The model under review builds one solid part; all positions refer to its coordinate system, in mm. A direction names the side the tool comes from. Round coordinates to 2 decimals unless told otherwise and drop trailing zeros. Write each loop counter-clockwise with the first axis right and the second up, starting at its lowest first coordinate (ties: lowest second). Pieces come first, ordered by that corner, then holes. Notation, with made-up numbers: (81, -20) - (103, -20) arc R11 cw to (103, -6) - close; hole circle Ø9 at (61, 79). An arc over 180 degrees is marked (long way). Write each question's results on one line, items separated by ' | '.
```python
from build123d import *

# Parameters (mm, degrees)
ESQUISSE1_R        = 76.15
ESQUISSE1_R_2      = 51.25
BOSS_EXTRU_1_DEPTH = 4
SKETCH1_R          = 1
AIR_VENTS_DEPTH    = 108.766622848
CUT_EXTRUDE1_DEPTH = 10


with BuildPart() as part:
    # Esquisse1 → Boss.-Extru.1 (new body)
    with BuildSketch(Plane(origin=(0, 0, 0), x_dir=(0, 0, -1), z_dir=(1, 0, 0))):
        Circle(ESQUISSE1_R)
        Circle(ESQUISSE1_R_2, mode=Mode.SUBTRACT)
    extrude(amount=BOSS_EXTRU_1_DEPTH)

    # Sketch1 → air vents (cut, through all)
    with BuildSketch(Plane(origin=(4, 0, 0), x_dir=(0, 0, -1), z_dir=(1, 0, 0))):
        with Locations((0, 60)):
            Circle(SKETCH1_R)
        with Locations((60, 0)):
            Circle(SKETCH1_R)
        with Locations((0, -60)):
            Circle(SKETCH1_R)
        with Locations((-60, 0)):
            Circle(SKETCH1_R)
    extrude(amount=-AIR_VENTS_DEPTH, mode=Mode.SUBTRACT)

    # Sketch2 → Cut-Extrude1 (cut)
    with BuildSketch(Plane(origin=(4, 0, 0), x_dir=(0, 0, -1), z_dir=(1, 0, 0))):
        with BuildLine():
            Line((-43.487067043, 52.679455198), (-81.600352415, 90.79274057))
            Line((-81.600352415, 90.79274057), (-92.273966974, 83.081578819))
            Line((-92.273966974, 83.081578819), (-52.679455198, 43.487067043))
            ThreePointArc((-52.679455198, 43.487067043), (-43.487067043, 43.487067043), (-43.487067043, 52.679455198))
        make_face()
    extrude(amount=-CUT_EXTRUDE1_DEPTH, mode=Mode.SUBTRACT)


solid = part.part
```
Q1. For probe 1 along Y at (x, z) = (2, 0); probe 2 along Z at (x, y) = (0.55, 21); probe 3 along Y at (x, z) = (0.7, 47), list the stretches that pass through material, from the lowest coordinate up.
Evaluation:
probe 1: y = -76.15 to -61, -59 to -51.25, 51.25 to 59, 61 to 76.15 | probe 2: z = -73.2 to -46.75, 46.75 to 73.2 | probe 3: y = -59.92 to -20.43, 20.43 to 41.67, 56.19 to 59.92
Q2. The part is to be moulded in two halves that separate along Y. For faces 1 (the flat face through (0, -16, -50)), 2 (the cylindrical face through (1.97, -50.03, 11.11)), 3 (the flat face through (2.03, 46.31, 55.5)), say which applies: released by +Y, released by -Y, zero draft, split by the parting line, or undercut.
Evaluation:
face 1: zero draft | face 2: undercut | face 3: released by +Y
Q3. We need section A-A (x = 3). State the section outline as (y, z) points.
Evaluation:
outline: (43.49, 52.68) - (49.05, 58.25) arc R76.15 ccw (long way) to (58.25, 49.05) - (52.68, 43.49) arc R6.5 cw to start; hole circle Ø2 at (-60, 0); hole circle Ø102.5 at (0, 0); hole circle Ø2 at (0, -60); hole circle Ø2 at (0, 60); hole circle Ø2 at (60, 0)
Q4. Insertion check: P1, Ø5, axis at y = 31.5, z = 34, coming from the -X side; P2, Ø1, axis at x = 2.5, y = -57, coming from the +Z side; P3, Ø10, axis at y = -33.5, z = -34.5, coming from the -X side; P4, Ø1.5, axis at x = 3, z = 1.5, coming from the -Y side. Each pin has a flat end and moves straight along its axis. Give the tip position at first contact, or say it passes through.
Evaluation:
P1: passes through | P2: stops at z = 51.05 | P3: stops at x = 0 | P4: stops at y = -76.15
Q5. We need section B-B (y = 18.5). State the section outline as (x, z) points, plus the area to 3 significant figures.
Evaluation:
outline: (0, -73.87) - (4, -73.87) - (4, -47.79) - (0, -47.79) - close; (0, 47.79) - (4, 47.79) - (4, 73.87) - (0, 73.87) - close | area: 209 mm^2
Q6. We need section D-D (y = 55). State the section outline as (x, z) points, plus the area to 3 significant figures.
Evaluation:
outline: (0, -52.67) - (4, -52.67) - (4, 45.81) - (0, 45.81) - close | area: 394 mm^2
Q7. Tool access review of faces 4 (the flat face through (4, -16, -50)), 5 (the flat face through (2.03, 55.42, 46.23)): name each direction out of +Z, -Z, +X, -X, +Y, -Y from which nothing blocks a thin tool from reaching the whole face with its end or side.
Evaluation:
face 4: +Z, -Z, +X, +Y, -Y | face 5: +Z, +X, -X
Q8. We need section C-C (z = 26). State the section outline as (x, y) points, plus the area to 3 significant figures.
Evaluation:
outline: (0, -71.57) - (4, -71.57) - (4, -44.17) - (0, -44.17) - close; (0, 44.17) - (4, 44.17) - (4, 71.57) - (0, 71.57) - close | area: 219 mm^2
